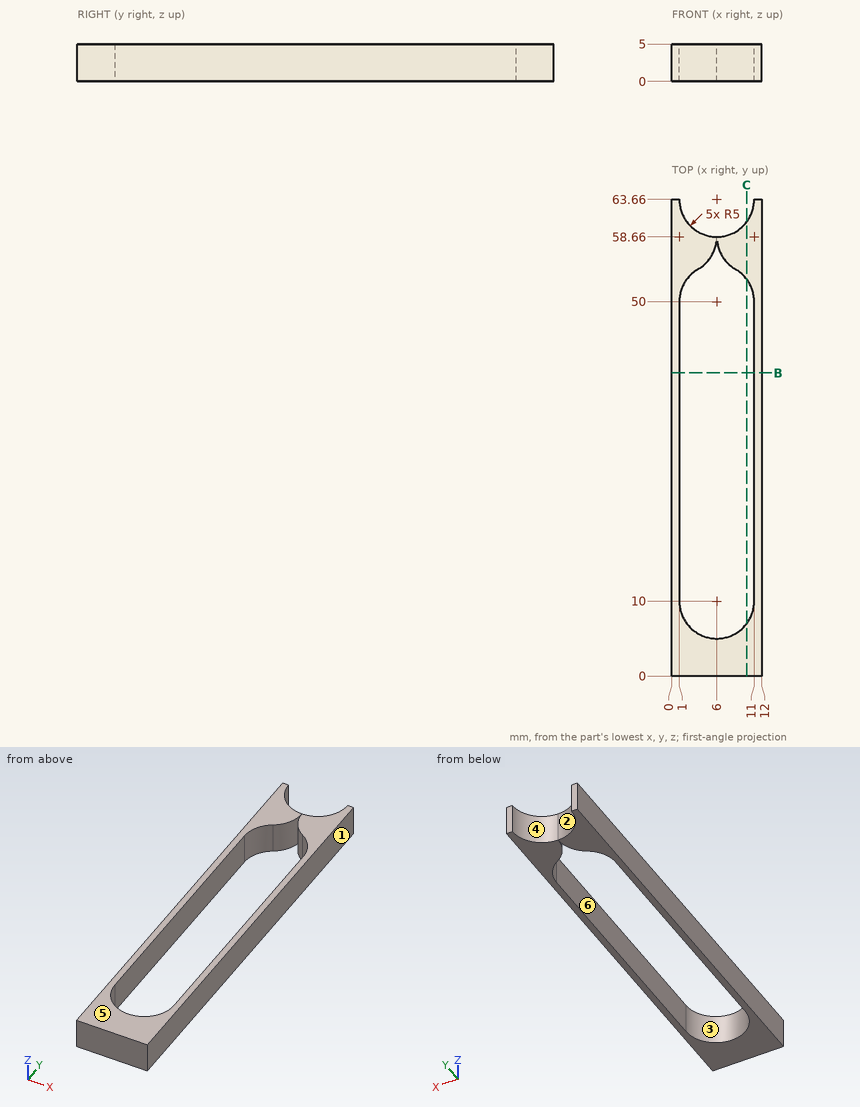
Study the drawing (mm; zero at the part's minimum x, y, z) and answer. A direction names the side the tool comes from. Coordinates: 2 decimals unless noted, no trailing zeros. Loops run counter-clockwise (first coordinate to the right, second up) from the corner with the lowest first, then second, coordinate; pieces in that order, holes last. Notation, with made-up numbers: M -24,61 L -9,61 A17 cw -9,75 Z; hole C -27.5,88 d4. An arc over 180 degrees is marked long. Answer as a JSON object with one key per item and string values. Group by question number.
Item 1: Determine the mould class of the marked faces 4, 5 and 6 for opening direction Y: +Y half, -Y half, draft (parallel to the pull), parting line (faces both ways), or undercut.
Item 2: Section C-C (x = 10) is taken. Write down the section's boundary in (y, z).
Item 3: This flat-tipped pin is pushed along its axis until it touches: P1, Ø6, axis at x = 5, y = 24, coming from the -Z side. Where does it stop, or does it pass through?
Item 4: Section B-B (y = 40.5) is taken. Write down the section's boundary in (x, z), and give its area (3 significant figures).
Item 5: Which of the six approach directions +Z, -Z, +X, -X, +Y, -Y give full straight-line access (tool end or side, diameter ignored) to the marked faces 1, 2 and 3?
Item 6: Consider L1, parallel to X at y = 32, z = 2.9; L2, parallel to Y at x = 5.5, z = 3.1 (1 decimal); L3, parallel to Y at x = 8.25, z = 3.8 (1 decimal). Determine where each line is inside the solid, lowest interval first.
Solved:
{
 "1": {"face 4": "+Y half", "face 5": "draft", "face 6": "undercut"},
 "2": {"outline": "M 0,0 L 7,0 L 7,5 L 0,5 Z; M 53,0 L 60.66,0 L 60.66,5 L 53,5 Z"},
 "3": {"P1": "passes through"},
 "4": {"outline": "M 0,0 L 1,0 L 1,5 L 0,5 Z; M 11,0 L 12,0 L 12,5 L 11,5 Z", "area": "10.0 mm2"},
 "5": {"face 1": "+Z, -Z, +X, +Y, -Y", "face 2": "+Z, -Z, +Y", "face 3": "+Z, -Z"},
 "6": {"L1": "x = 0 to 1, 11 to 12", "L2": "y = 0 to 5, 56.5 to 58.7", "L3": "y = 0 to 5.5, 54.5 to 59.2"}
}
